Geometry check sheet. Reference: the model listing, model coordinates, mm. Face numbers are marked on the shaded views. A direction names the side the tool comes from. Round coordinates to 2 decimals unless told otherwise and drop trailing zeros. Order: outer loops, then holes, each group sorted by start corner. A loop starts at its lowest first (then second) coordinate and runs counter-clockwise, first axis right, second up. Notation, with made-up numbers: (42, 55) -> (67, 55) arc R23 ccw to (67, 68) -> close; hole circle Ø6 at (79, 84). An arc over 180 degrees is marked (long way). Use a Markdown table: item, result. Add a question column.
Item 1: Material ranges on probe 1 along Z at (x, y) = (-47.5, 2.55); probe 2 along Z at (x, y) = (-30, 1.8); probe 3 along X at (y, z) = (1.15, 10), recorded low to high. Write a range as [from, to].
Item 2: Sectioned sample at A-A, the plane x = -47.5. Record the cut outline in (y, z), and give its area (3 significant figures).
Item 3: Gauge pin test, flat ends, axial feed: pin 1 Ø3 at (x, z) = (47.5, -10) entering from +Y; pin 2 Ø12 at (x, z) = (-6.5, -7.5) entering from +Y; pin 3 Ø3 at (x, z) = (-1.5, 6.5) entering from +Y. Record the tip position at first contact, or that the pin passes through.
Item 4: Sectioned sample at C-C, the plane x = -30. Record the cut outline in (y, z).
Item 5: Set-up check for the marked faces 1 and 2: record each of +Z, -Z, +X, -X, +Y, -Y from which the full face is reachable in a straight line by a thin tool's end or side.
Item 6: Sectioned sample at B-B, the plane z = -10. Record the cut outline in (x, y), and give its area (3 significant figures).
Item 7: Sectioned sample at D-D, the plane z = -5.25. Record the cut outline in (x, y).
from build123d import *

# Parameters (mm, degrees)
SKETCH1_W                                    = 110
SKETCH1_H                                    = 30
EXTRUDE1_DEPTH                               = 3
CUT_EXTRUDE1_DEPTH                           = 58.087651905
CHAMFER1_SIZE                                = 9
CHAMFER1_SIZE2                               = 2.5
CSK_FOR_M3_COUNTERSUNK_RAISED_HEAD_S_2_COUNT = 2
CSK_FOR_M3_COUNTERSUNK_RAISED_HEAD_S_2_PITCH = 95
CSK_FOR_M3_COUNTERSUNK_RAISED_HEAD_S_3_COUNT = 2
CSK_FOR_M3_COUNTERSUNK_RAISED_HEAD_S_3_PITCH = 97.082439195
CSK_FOR_M3_COUNTERSUNK_RAISED_HEAD_S_4_COUNT = 2
CSK_FOR_M3_COUNTERSUNK_RAISED_HEAD_S_4_PITCH = 20
M3_TAPPED_HOLE1_D                            = 3


with BuildPart() as part:
    # Sketch1 → Extrude1 (new body)
    with BuildSketch(Plane(origin=(0, 0, 0), x_dir=(1, 0, 0), z_dir=(0, 1, 0))):
        Rectangle(SKETCH1_W, SKETCH1_H)
    extrude(amount=EXTRUDE1_DEPTH)

    # Sketch2 → Cut-Extrude1 (cut, through all)
    with BuildSketch(Plane(origin=(0, 3, 0), x_dir=(-1, 0, 0), z_dir=(0, 1, 0))):
        with BuildLine():
            Line((5, 0), (5, -15))
            Line((5, -15), (-5, -15))
            Line((-5, -15), (-5, 0))
            ThreePointArc((-5, 0), (0, 5), (5, 0))
        make_face()
    extrude(amount=-CUT_EXTRUDE1_DEPTH, mode=Mode.SUBTRACT)

    # Chamfer1
    chamfer1_edges = [part.edges().sort_by_distance(p)[0] for p in [
        (0, 3, 5),
        (5, 3, -7.5),
        (-5, 3, -7.5),
    ]]
    chamfer1_side = [part.faces().sort_by_distance(p)[0] for p in [
        (-53.859824575, 3, 0),
    ]]
    chamfer(chamfer1_edges, length=CHAMFER1_SIZE, length2=CHAMFER1_SIZE2, reference=chamfer1_side[0])

    # Sketch8 → CSK for M3 Countersunk Raised Head Screw1 (revolve, cut)
    with BuildSketch(Plane(origin=(47.5, 0, -10), x_dir=(0, 0, -1), z_dir=(1, 0, 0))):
        Polygon((0, 0), (0, 3), (1.7, 3), (1.7, 1.45), (3.15, 0), align=None)
    csk_for_m3_countersunk_raised_head_screw = revolve(axis=Axis((47.5, -6.35, -10), (0, 1, 0)), mode=Mode.SUBTRACT)

    # CSK for M3 Countersunk Raised Head S 2: CSK for M3 Countersunk Raised Head Screw1 ×2
    with Locations(*[(-i * CSK_FOR_M3_COUNTERSUNK_RAISED_HEAD_S_2_PITCH, 0, 0) for i in range(1, CSK_FOR_M3_COUNTERSUNK_RAISED_HEAD_S_2_COUNT)]):
        add(csk_for_m3_countersunk_raised_head_screw, mode=Mode.SUBTRACT)

    # CSK for M3 Countersunk Raised Head S 3: CSK for M3 Countersunk Raised Head Screw1 ×2
    with Locations(*[Vector(-0.978549784986749, 0, 0.20601048104984188) * (i * CSK_FOR_M3_COUNTERSUNK_RAISED_HEAD_S_3_PITCH) for i in range(1, CSK_FOR_M3_COUNTERSUNK_RAISED_HEAD_S_3_COUNT)]):
        add(csk_for_m3_countersunk_raised_head_screw, mode=Mode.SUBTRACT)

    # CSK for M3 Countersunk Raised Head S 4: CSK for M3 Countersunk Raised Head Screw1 ×2
    with Locations(*[(0, 0, i * CSK_FOR_M3_COUNTERSUNK_RAISED_HEAD_S_4_PITCH) for i in range(1, CSK_FOR_M3_COUNTERSUNK_RAISED_HEAD_S_4_COUNT)]):
        add(csk_for_m3_countersunk_raised_head_screw, mode=Mode.SUBTRACT)

    # M3 Tapped Hole1 (through all)
    with Locations(Plane(origin=(0, 3, 0), x_dir=(-1, 0, 0), z_dir=(0, 1, 0))):
        with Locations((-30, 0), (30, 0)):
            Hole(M3_TAPPED_HOLE1_D / 2)


solid = part.part
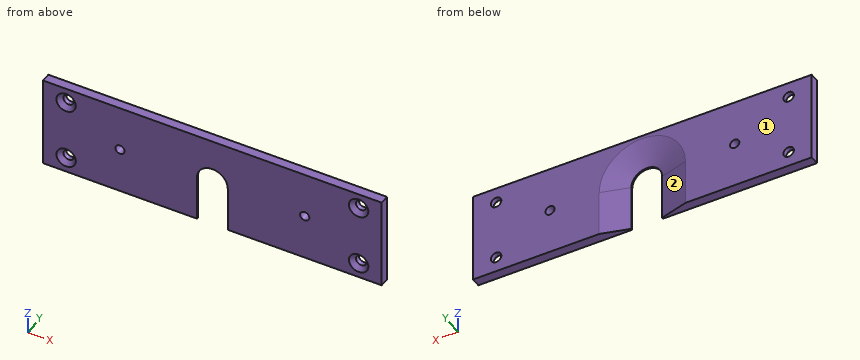
Found:
| question | item | result |
|---|---|---|
| 1 | probe 1 | z = [-15, -11.7], [-8.3, 8.3], [11.7, 15] |
| 1 | probe 2 | z = [-15, -1.5], [1.5, 15] |
| 1 | probe 3 | x = [-55, -49.5], [-45.5, 45.5], [49.5, 55] |
| 2 | outline | (0, -15) -> (3, -15) -> (3, -11.7) -> (1.45, -11.7) -> (0, -13.15) -> close; (0, -6.85) -> (1.45, -8.3) -> (3, -8.3) -> (3, 8.3) -> (1.45, 8.3) -> (0, 6.85) -> close; (0, 13.15) -> (1.45, 11.7) -> (3, 11.7) -> (3, 15) -> (0, 15) -> close |
| 2 | area | 65.4 mm2 |
| 3 | pin 1 | passes through |
| 3 | pin 2 | stops at y = 2.58 |
| 3 | pin 3 | stops at y = 1.38 |
| 4 | outline | (0, -15) -> (3, -15) -> (3, -1.5) -> (0, -1.5) -> close; (0, 1.5) -> (3, 1.5) -> (3, 15) -> (0, 15) -> close |
| 5 | face 1 | +Z, -Z, +X, -X, +Y |
| 5 | face 2 | -Z, +Y |
| 6 | outline | (-55, 0) -> (-50.65, 0) -> (-49.2, 1.45) -> (-49.2, 3) -> (-55, 3) -> close; (-45.8, 1.45) -> (-44.35, 0) -> (-5, 0) -> (-5, 0.5) -> (-14, 3) -> (-45.8, 3) -> close; (5, 0) -> (44.35, 0) -> (45.8, 1.45) -> (45.8, 3) -> (14, 3) -> (5, 0.5) -> close; (49.2, 1.45) -> (50.65, 0) -> (55, 0) -> (55, 3) -> (49.2, 3) -> close |
| 6 | area | 253 mm2 |
| 7 | outline | (-55, 0) -> (-5, 0) -> (-5, 0.5) -> (-14, 3) -> (-55, 3) -> close; (5, 0) -> (55, 0) -> (55, 3) -> (14, 3) -> (5, 0.5) -> close |
